Check sheet for the modelled part. Datum: model origin and axes. Units: mm. A direction names the side the tool comes from. Coordinates: 2 decimals unless noted, no trailing zeros. Loops run counter-clockwise (first coordinate to the right, second up) from the corner with the lowest first, then second, coordinate; pieces in that order, holes last.
from build123d import *

# Parameters (mm, degrees)
SKETCH1_R           = 4
BOSS_EXTRUDE1_DEPTH = 5
SKETCH2_W           = 29.745771512
SKETCH2_H           = 31.069071225
CUT_EXTRUDE1_DEPTH  = 22.477415783
SKETCH3_W           = 10
SKETCH3_H           = 15
BOSS_EXTRUDE2_DEPTH = 10
FILLET1_R           = 13
FILLET2_R           = 5
FILLET3_R           = 2
FILLET4_R           = 2
SKETCH4_R           = 2.5
CUT_EXTRUDE2_DEPTH  = 7
SKETCH6_W           = 5.480044722
SKETCH6_H           = 16.421651107
CUT_EXTRUDE3_DEPTH  = 52.045615162


with BuildPart() as part:
    # Sketch1 → Boss-Extrude1 (new body)
    with BuildSketch(Plane.XY):
        with BuildLine():
            Line((-22.23071963, 10.602474367), (22.76928037, 9.390273126))
            ThreePointArc((22.76928037, 9.390273126), (32.496373747, -0.875380991), (22.23071963, -10.602474367))
            Line((22.23071963, -10.602474367), (-22.76928037, -9.390273126))
            ThreePointArc((-22.76928037, -9.390273126), (-32.496373747, 0.875380991), (-22.23071963, 10.602474367))
        make_face()
        with Locations((22.5, -0.606100621)):
            Circle(SKETCH1_R, mode=Mode.SUBTRACT)
        with Locations((-22.5, 0.606100621)):
            Circle(SKETCH1_R, mode=Mode.SUBTRACT)
    extrude(amount=BOSS_EXTRUDE1_DEPTH)

    # Sketch2 → Cut-Extrude1 (cut, through all)
    with BuildSketch(Plane(origin=(0.26928037, 9.996373747, 0), x_dir=(0.999637375, -0.026928037, 0), z_dir=(0.026928037, 0.999637375, 0))):
        with Locations((27.899171519, 0.562166988)):
            Rectangle(SKETCH2_W, SKETCH2_H)
    extrude(amount=-CUT_EXTRUDE1_DEPTH, mode=Mode.SUBTRACT)

    # Sketch3 → Boss-Extrude2 (add)
    with BuildSketch(Plane(origin=(0.26928037, 9.996373747, 0), x_dir=(0.999637375, -0.026928037, 0), z_dir=(0.026928037, 0.999637375, 0))):
        with Locations((13.026285763, -2.5)):
            Rectangle(SKETCH3_W, SKETCH3_H)
    extrude(amount=BOSS_EXTRUDE2_DEPTH)

    # Fillet1
    fillet1_edges = [part.edges().sort_by_distance(p)[0] for p in [
        (12.752281732, -10.347146052, 2.5),
    ]]
    fillet(fillet1_edges, radius=FILLET1_R)

    # Fillet2
    fillet2_edges = [part.edges().sort_by_distance(p)[0] for p in [
        (8.292655599, 9.780241626, 2.5),
    ]]
    fillet(fillet2_edges, radius=FILLET2_R)

    # Fillet3
    fillet3_edges = [part.edges().sort_by_distance(p)[0] for p in [
        (10.791749036, 9.712921534, 0),
        (10.791749036, 9.712921534, 5),
        (13.290842472, 9.645601441, 2.5),
        (8.359975692, 12.279335063, 0),
        (8.359975692, 12.279335063, 5),
    ]]
    fillet(fillet3_edges, radius=FILLET3_R)

    # Fillet4
    fillet4_edges = [part.edges().sort_by_distance(p)[0] for p in [
        (8.427295784, 14.7784285, -5),
        (8.427295784, 14.7784285, 10),
        (18.289029346, 9.510961256, 2.5),
        (18.423669531, 14.509148129, 10),
        (18.423669531, 14.509148129, -5),
        (8.561935969, 19.776615373, 2.5),
        (13.560122843, 19.641975188, 10),
        (18.558309716, 19.507335003, 2.5),
        (13.560122843, 19.641975188, -5),
    ]]
    fillet(fillet4_edges, radius=FILLET4_R)

    # Sketch4 → Cut-Extrude2 (cut)
    with BuildSketch(Plane(origin=(0.538560741, 19.992747493, 0), x_dir=(0.999637375, -0.026928037, 0), z_dir=(0.026928037, 0.999637375, 0))):
        with Locations((13.026285763, -2.5)):
            Circle(SKETCH4_R)
    extrude(amount=-CUT_EXTRUDE2_DEPTH, mode=Mode.SUBTRACT)

    # Sketch6 → Cut-Extrude3 (cut, through all)
    with BuildSketch(Plane(origin=(18.019748975, -0.485412491, 0), x_dir=(0, 0, -1), z_dir=(0.999637375, -0.026928037, 0))):
        with Locations((4.740022361, 14.542229601)):
            Rectangle(SKETCH6_W, SKETCH6_H)
        with Locations((-9.740022361, 14.542229601)):
            Rectangle(SKETCH6_W, SKETCH6_H)
    extrude(amount=-CUT_EXTRUDE3_DEPTH, mode=Mode.SUBTRACT)


solid = part.part
(1) Section check A-A, the plane z = 1.5. Enter the section's corners in (x, y).
(2) Section check B-B, the plane z = 6. Enter the section's corners in (x, y), plus the area to 3 significant figures.
(3) Scan lines: line 1 along Y through (x, z) = (-22.5, 2.1); line 2 along Z through (x, y) = (-5, 9.5); line 3 along X through (y, z) = (-1, 2.5). Record each from-to range of solid material in increasing order.
(4) Section check D-D, the plane x = -12. Enter the section's corners in (y, z).
(5) Set-up check for faces 1 (the face through (7.939, 10.561, 5.835)), 2 (the face through (7.41, 11.89, 2.44)), 3 (the face through (13, 15, -2)): record each of +Z, -Z, +X, -X, +Y, -Y from which the full face is reachable in a straight line by a thin tool's end or side.
(6) Draft check along Y on faces 4 (the face through (9.15, 19.19, 2.44)), 5 (the face through (11.484, 16.246, 4.021)), 6 (the face through (14.15, 9.27, 2.44)). Enter one of: pulls with the +Y half, pulls with the -Y half, needs draft (parallel to the pull), parting line crosses it, or undercut.
(7) Gauge pin test, flat ends, axial feed: P1, Ø1, axis at y = 4, z = 1.5, coming from the +X side; P2, Ø1.5, axis at x = -12, y = -2.5, coming from the +Z side; P3, Ø8, axis at x = 1.5, y = 5, coming from the -Z side. Record the tip position at first contact, or that the pin passes through.
(8) Section check C-C, the plane y = -6.25. Enter the section's corners in (x, z).
Determined:
1. outline: (-22.77, -9.39) - (-0.24, -10) arc R13 ccw to (13.1, 2.65) - (13.24, 7.65) arc R2 cw to (15.29, 9.59) - (16.29, 9.56) arc R2 ccw to (18.34, 11.51) - (18.5, 17.51) arc R2 ccw to (16.56, 19.56) - (15.85, 19.58) - (15.66, 12.58) - (11.08, 12.71) - (11.27, 19.7) - (10.56, 19.72) arc R2 ccw to (8.51, 17.78) - (8.43, 14.78) arc R5 cw to (3.29, 9.91) - (-22.23, 10.6) arc R10 ccw to start; hole circle Ø8 at (-22.5, 0.61)
2. outline: (8.02, 9.52) - (14.28, 9.35) arc R2 cw to (15.29, 9.59) - (16.29, 9.56) arc R2 ccw to (18.34, 11.51) - (18.5, 17.51) arc R2 ccw to (16.56, 19.56) - (10.56, 19.72) arc R2 ccw to (8.51, 17.78) - (8.43, 14.78) arc R5 cw to (8.12, 13.17) - close
2. area: 100 mm2
3. line 1: y = -9.4 to -3.39, 4.61 to 10.61
3. line 2: z = 0 to 5
3. line 3: x = -32.37 to -26.16, -18.84 to 12.48
4. outline: (-9.68, 0) - (10.33, 0) - (10.33, 5) - (-9.68, 5) - close
5. face 1: +Z, -X, +Y
5. face 2: +Z, -Z, +Y
5. face 3: -Z, +X, -X, +Y, -Y
6. face 4: pulls with the +Y half
6. face 5: undercut
6. face 6: pulls with the -Y half
7. P1: stops at x = 13.15
7. P2: stops at z = 5
7. P3: stops at z = 0
8. outline: (-29.78, 0) - (9.24, 0) - (9.24, 5) - (-29.78, 5) - close
